Design review of the part built by this model. Coordinates are the model's own, in mm. A direction names the side the tool comes from. Coordinates: 2 decimals unless noted, no trailing zeros. Write each loop counter-clockwise with the first axis right and the second up, starting at its lowest first coordinate (ties: lowest second). Pieces come first, ordered by that corner, then holes.
Q1. Clearance check with flat-ended pins moving along their axes: pin 1 Ø12 at (y, z) = (-29.5, 6) entering from +X; pin 2 Ø0.6 at (x, z) = (-33, 0) entering from -Y; pin 3 Ø11 at (x, y) = (-21.5, 14.5) entering from +Z; pin 4 Ø12 at (x, z) = (-12, -9.5) entering from +Y. State where each tip first meets the part, or that it passes through.
Q2. Machinability: for faces 4 (the face through (-22, 12, -1)), 5 (the face through (-22.56, -0.15, 7.5)), 6 (the face through (-32.78, -37.45, 2.34)), 7 (the face through (-33.123, 0.05, -37.316)), which of the approach directions +Z, -Z, +X, -X, +Y, -Y give a long, thin tool a straight path to every point of the face, cutting with its end or side? Answer none if there is none.
Q3. Add section D-D, the plane x = -6. Give the boundary of the cut face in (y, z).
Q4. Add section B-B, the plane x = -15. Give the boundary of the cut face in (y, z).
Q5. To check wall thickness, follow probe 1 along Z at (x, y) = (-28.5, 0.5); probe 2 along Z at (x, y) = (-10.5, -36); probe 3 along Y at (x, z) = (-13, -33). State the ranges of each line that lie inside material, in increasing order.
Q6. The part is to be moulded in two halves that separate along Z. For faces 1 (the face through (-26.88, 39.09, -1.71)), 2 (the face through (-33.123, -0.05, 37.316)), 3 (the face through (-21.94, 6.78, -6.86)), say which applies: +Z half, -Z half, draft (parallel to the pull), parting line (faces both ways), or undercut.
Q7. Add section C-C, the plane x = -41. Give the boundary of the cut face in (y, z).
Q8. Add section A-A, the plane y = 0. Give the boundary of the cut face in (x, z), plus the area to 3 significant figures.
Autodesk Inventor part; units mm, degrees
ref_plane "YZ Plane" through (0, 0, 0) normal (1, 0, 0) x (0, 1, 0)
ref_plane "XZ Plane" through (0, 0, 0) normal (0, 1, 0) x (-1, 0, 0)
ref_plane "XY Plane" through (0, 0, 0) normal (0, 0, 1) x (1, 0, 0)
sketch "Esquisse1" plane through (0, 0, 0) normal (0, 0, 1) x (1, 0, 0)
  line L0 (-36.1898, 0) -> (37.2521, 0)
  line L1 (0, 7.5) -> (-44.5, 7.5)
  line L2 (-44.5, 7.5) -> (-44.5, 36.75)
  line L3 (-44.5, 36.75) -> (0, 42.75)
  line L4 (0, 42.75) -> (0, 7.5)
  point P0 (0, 0)
  dimension "d0" = 15
  dimension "d1" = 85.5
  dimension "d2" = 0
  dimension "d3" = 73.5
  dimension "d4" = 44.5
  dimension "d5" = 0
revolve "Révolution1" add sketch "Esquisse1" angle 360 about axis through (-36.1898, 0, 0) along (1, 0, 0)
sketch "Esquisse3" plane through (0, 0, 0) normal (1, 0, 0) x (0, 0, -1)
  circle A0 centre (0, 0) radius 41
  circle A1 centre (0, 0) radius 7.5
  line L0 (0, 0) -> (-59.2945, 0)
  line L1 (0, 0) -> (0, -53.2291)
  line L2 (0, 0) -> (55.0659, 0)
  point P0 (0, -41)
  point P1 (41, 0)
  point P2 (-41, 0)
  dimension "d16" = 82
hole "Perçage1" at (0, -41, 0) at (0, 0, 41) at (0, 0, -41) direction (-1, 0, 0) diameter 10.106 depth 32.3 tip angle 118
sketch "Esquisse4" plane through (0, 0, 0) normal (1, 0, 0) x (0, 0, 1)
  line L0 (0, 0) -> (-39.036, -39.036)
  line L1 (0, 0) -> (-55.3193, 0)
  circle A0 centre (0, 0) radius 7.5
  line L2 (-1.6577, -7.3145) -> (-3.9911, -9.648)
  line L3 (-7.3145, -1.6577) -> (-9.648, -3.9911)
  line L4 (-9.648, -3.9911) -> (-3.9911, -9.648)
  dimension "d17" = 45
  dimension "d20" = 3.3
  dimension "d21" = 3.3
  dimension "d22" = 4
  dimension "d23" = 4
extrude "Extrusion1" cut sketch "Esquisse4" against normal through all contours A0 L2 L4 L0 | L0 L4 L3 A0
sketch "Esquisse5" plane through (0, 0, 0) normal (1, 0, 0) x (0, 0, 1)
  line L0 (-1, 42.75) -> (1, 42.75)
  line L1 (1, 42.75) -> (1, -17.25)
  line L2 (1, -17.25) -> (-1, -17.25)
  line L3 (-1, -17.25) -> (-1, 42.75)
  line L4 (-1, 42.75) -> (1, -17.25) construction
  line L5 (1, 42.75) -> (-1, -17.25) construction
  arc A0 (-4.8326, 42.476) -> (4.8326, 42.476) centre (0, 0) ccw
  point P0 (0, 12.75)
  point P1 (42.6948, 2.1722)
  point P2 (-42.6948, 2.1722)
  point P3 (4.9266, -42.4652)
  point P4 (42.5102, -4.5219)
  dimension "d26" = 2
  dimension "d27" = 60
  dimension "d28" = 0
extrude "Extrusion2" cut sketch "Esquisse5" against normal through all
properties part number "Douille2517"
Here are the results:
1. pin 1: stops at x = 0
1. pin 2: stops at y = 17.25
1. pin 3: stops at z = 39.03
1. pin 4: stops at y = 41.37
2. face 4: +X, -X, -Y
2. face 5: +X, -X
2. face 6: +X, -Y
2. face 7: -Z, +X
3. outline: (-41.64, -5.01) arc R41.94 ccw to (-5.01, -41.64) arc R5.05 cw (long way) to (5.01, -41.64) arc R41.94 ccw to (5.01, 41.64) arc R5.05 cw (long way) to (-5.01, 41.64) arc R41.94 ccw to (-41.64, 5.01) arc R5.05 cw to (-36.05, 1) - (-7.43, 1) arc R7.5 cw to (7.43, 1) - (17.25, 1) - (17.25, -1) - (7.43, -1) arc R7.5 cw to (7.31, -1.66) - (9.65, -3.99) - (3.99, -9.65) - (1.66, -7.31) arc R7.5 cw to (-7.43, -1) - (-36.05, -1) arc R5.05 cw to start
4. outline: (-40.42, -5.02) arc R40.73 ccw to (-5.02, -40.42) arc R5.05 cw to (5.02, -40.42) arc R40.73 ccw to (5.02, 40.42) arc R5.05 cw to (-5.02, 40.42) arc R40.73 ccw to (-40.42, 5.02) arc R5.05 cw to (-36.05, 1) - (-7.43, 1) arc R7.5 cw to (7.43, 1) - (17.25, 1) - (17.25, -1) - (7.43, -1) arc R7.5 cw to (7.31, -1.66) - (9.65, -3.99) - (3.99, -9.65) - (1.66, -7.31) arc R7.5 cw to (-7.43, -1) - (-36.05, -1) arc R5.05 cw to start
5. probe 1: z = -35.97 to -7.48, 7.48 to 35.97
5. probe 2: z = -20.31 to -1, 1 to 20.31
5. probe 3: y = -24.33 to 24.33
6. face 1: parting line
6. face 2: +Z half
6. face 3: undercut
7. outline: (-37.21, -1) arc R37.22 ccw (long way) to (-37.21, 1) - (-7.43, 1) arc R7.5 cw to (7.43, 1) - (17.25, 1) - (17.25, -1) - (7.43, -1) arc R7.5 cw to (7.31, -1.66) - (9.65, -3.99) - (3.99, -9.65) - (1.66, -7.31) arc R7.5 cw to (-7.43, -1) - close
8. outline: (-44.5, -36.75) - (-33.66, -38.21) - (-32.3, -35.95) - (0, -35.95) - (0, -7.5) - (-44.5, -7.5) - close; (-44.5, 7.5) - (0, 7.5) - (0, 35.95) - (-32.3, 35.95) - (-33.66, 38.21) - (-44.5, 36.75) - close
8. area: 2,570 mm2
